Could you check a few things on this model? Use its own coordinates, in mm. A direction names the side the tool comes from. Round coordinates to 2 decimals unless told otherwise and drop trailing zeros. Write each loop counter-clockwise with the first axis right and the second up, starting at its lowest first coordinate (ties: lowest second). Pieces come first, ordered by that corner, then holes. Notation, with made-up numbers: (38.5, 12) - (54.5, 12) arc R18 ccw to (54.5, 44) - close; hole circle Ø8 at (28, -17.5). An arc over 180 degrees is marked (long way). Put each result on its own line as item: value.
from build123d import *

# Parameters (mm, degrees)
BOSS_EXTRUDE1_DEPTH = 11
CHAMFER4_SIZE       = 1
CHAMFER5_SIZE       = 1


with BuildPart() as part:
    # Sketch1 → Boss-Extrude1 (new body)
    with BuildSketch(Plane(origin=(0, 0, 0), x_dir=(0, 0, -1), z_dir=(1, 0, 0))):
        with BuildLine():
            Line((28, 1.391885412), (-28, 1.391885412))
            Line((-28, 1.391885412), (-29.5, 2.257910816))
            ThreePointArc((-29.5, 2.257910816), (-30.866025404, 1.891885412), (-30.5, 0.525860008))
            Line((-30.5, 0.525860008), (-30, 0.237184874))
            Line((-30, 0.237184874), (-30, -9.608114588))
            Line((-30, -9.608114588), (-40, -9.608114588))
            Line((-40, -9.608114588), (-40, 1.391885412))
            Line((-40, 1.391885412), (-19, 88.391885412))
            Line((-19, 88.391885412), (-9, 88.391885412))
            Line((-9, 88.391885412), (-9, 17.54658595))
            Line((-9, 17.54658595), (-9.5, 17.257910816))
            ThreePointArc((-9.5, 17.257910816), (-9.866025404, 15.891885412), (-8.5, 15.525860008))
            Line((-8.5, 15.525860008), (-7, 16.391885412))
            Line((-7, 16.391885412), (7, 16.391885412))
            Line((7, 16.391885412), (8.5, 15.525860008))
            ThreePointArc((8.5, 15.525860008), (9.866025404, 15.891885412), (9.5, 17.257910816))
            Line((9.5, 17.257910816), (9, 17.54658595))
            Line((9, 17.54658595), (9, 88.391885412))
            Line((9, 88.391885412), (19, 88.391885412))
            Line((19, 88.391885412), (40, 1.391885412))
            Line((40, 1.391885412), (40, -9.608114588))
            Line((40, -9.608114588), (30, -9.608114588))
            Line((30, -9.608114588), (30, 0.237184874))
            Line((30, 0.237184874), (30.5, 0.525860008))
            ThreePointArc((30.5, 0.525860008), (30.866025404, 1.891885412), (29.5, 2.257910816))
            Line((29.5, 2.257910816), (28, 1.391885412))
        make_face()
    extrude(amount=BOSS_EXTRUDE1_DEPTH)

    # Chamfer4
    chamfer4_edges = [part.edges().sort_by_distance(p)[0] for p in [
        (0, -4.685464857, 30),
        (11, -4.685464857, 30),
    ]]
    chamfer(chamfer4_edges, length=CHAMFER4_SIZE - 0.0001)  # a hair under: the kernel refuses the full size

    # Chamfer5
    chamfer5_edges = [part.edges().sort_by_distance(p)[0] for p in [
        (0, -4.685464857, -30),
        (11, -4.685464857, -30),
    ]]
    chamfer(chamfer5_edges, length=CHAMFER5_SIZE - 0.0001)  # a hair under: the kernel refuses the full size


solid = part.part
(1) Imagine slicing it at D-D, the plane z = -12.5. List the corners of the cut face in (x, y) for me, then the cut area to 3 significant figures.
Values found:
outline: (0, 1.39) - (11, 1.39) - (11, 88.39) - (0, 88.39) - close
area: 957 mm^2
(2) For faces 1 (the face through (5, -5, -30)), 2 (the face through (0, 40.1, -9.4)), 3 (the face through (5, 16.392, 0)), which set-ups out of +Z, -Z, +X, -X, +Y, -Y let a thin tool reach every point of the face, with its end or its side?
Values found:
face 1: +X, -X, -Y
face 2: +Z, -Z, -X, +Y, -Y
face 3: +X, -X, +Y
(3) Imagine slicing it at B-B, the plane x = 8.75. List the corners of the cut face in (y, z) for me, then the cut area to 3 significant figures.
Values found:
outline: (-9.61, -40) - (1.39, -40) - (88.39, -19) - (88.39, -9) - (17.55, -9) - (17.26, -9.5) arc R1 cw to (15.53, -8.5) - (16.39, -7) - (16.39, 7) - (15.53, 8.5) arc R1 cw to (17.26, 9.5) - (17.55, 9) - (88.39, 9) - (88.39, 19) - (1.39, 40) - (-9.61, 40) - (-9.61, 30) - (0.24, 30) - (0.53, 30.5) arc R1 cw to (2.26, 29.5) - (1.39, 28) - (1.39, -28) - (2.26, -29.5) arc R1 cw to (0.53, -30.5) - (0.24, -30) - (-9.61, -30) - close
area: 4,050 mm^2
(4) Imagine slicing it at A-A, the plane y = -2.5. List the corners of the cut face in (x, z) for me, then the cut area to 3 significant figures.
Values found:
outline: (0, -40) - (11, -40) - (11, -31) - (10, -30) - (1, -30) - (0, -31) - close; (0, 31) - (1, 30) - (10, 30) - (11, 31) - (11, 40) - (0, 40) - close
area: 218 mm^2
(5) If we mould it in two halves opening along Z, with no side actions, what happens to faces 4 (the face through (5, 88.392, -14)), 5 (the face through (5, 1.392, 0)), 6 (the face through (5.423, 45.501, -29.353)), 7 (the face through (5.423, 44.283, 29.647))? For each: pulls with the +Z half, pulls with the -Z half, needs draft (parallel to the pull), parting line crosses it, or undercut.
Values found:
face 4: needs draft
face 5: undercut
face 6: pulls with the -Z half
face 7: pulls with the +Z half
(6) Imagine slicing it at C-C, the plane y = 72. List the corners of the cut face in (x, z) for me, then the cut area to 3 significant figures.
Values found:
outline: (0, -22.96) - (11, -22.96) - (11, -9) - (0, -9) - close; (0, 9) - (11, 9) - (11, 22.96) - (0, 22.96) - close
area: 307 mm^2
(7) I'm going to push flat-ended pins straight in: pin 1 (4 mm diameter, centred on x = 7.5, y = 54, fed in from -Z); pin 2 (5.5 mm diameter, centred on x = 3.5, y = 62, fed in from -Z); pin 3 (3 mm diameter, centred on x = 1.5, z = -17.5, fed in from -Y). Where does each tip first touch, or does it pass through?
Values found:
pin 1: stops at z = -27.78
pin 2: stops at z = -26.03
pin 3: stops at y = 1.39
(8) Please list where these lines run through material, in increasing order: probe 1 along Y at (x, z) = (8, -16.5); probe 2 along Z at (x, y) = (8, 55.5); probe 3 along Y at (x, z) = (9, 1). Write a range as from..to.
Values found:
probe 1: y = 1.39..88.39
probe 2: z = -26.94..-9, 9..26.94
probe 3: y = 1.39..16.39
